```python
from build123d import *

# Parameters (mm, degrees)
SKETCH1_W            = 60
SKETCH1_H            = 45
BOSS_EXTRUDE1_DEPTH  = 5
SKETCH3_R            = 5.5
SKETCH3_R_2          = 3.025
BOSS_EXTRUDE2_DEPTH  = 8
SKETCH4_W            = 12
SKETCH4_H            = 16
SKETCH4_R            = 2.55
BOSS_EXTRUDE3_DEPTH  = 5
FILLET1_R            = 4
M4_CLEARANCE_HOLE1_D = 4.5
MIRROR1_OUTLINE_R    = 2.25
MIRROR1_DEPTH        = 5


# Read off the part's stored shape, not the designer's step: Mirror1
with BuildPart() as part:
    # Sketch1 → Boss-Extrude1 (new body)
    with BuildSketch(Plane.XY):
        Rectangle(SKETCH1_W, SKETCH1_H)
    extrude(amount=BOSS_EXTRUDE1_DEPTH)

    # Sketch3 → Boss-Extrude2 (add)
    # profile 1 of 4: a face of its own
    with BuildSketch(Plane.XY.offset(5)):
        with Locations((-19.2405, 11.938)):
            Circle(SKETCH3_R)
        with Locations((-19.2405, 11.938)):
            Circle(SKETCH3_R_2, mode=Mode.SUBTRACT)
    # profile 2 of 4: a face of its own
    with BuildSketch(Plane.XY.offset(5)):
        with Locations((-19.2405, -11.938)):
            Circle(SKETCH3_R)
        with Locations((-19.2405, -11.938)):
            Circle(SKETCH3_R_2, mode=Mode.SUBTRACT)
    # profile 3 of 4: a face of its own
    with BuildSketch(Plane.XY.offset(5)):
        with Locations((19.2405, 11.938)):
            Circle(SKETCH3_R)
        with Locations((19.2405, 11.938)):
            Circle(SKETCH3_R_2, mode=Mode.SUBTRACT)
    # profile 4 of 4: a face of its own
    with BuildSketch(Plane.XY.offset(5)):
        with Locations((19.2405, -11.938)):
            Circle(SKETCH3_R)
        with Locations((19.2405, -11.938)):
            Circle(SKETCH3_R_2, mode=Mode.SUBTRACT)
    extrude(amount=BOSS_EXTRUDE2_DEPTH)

    # Sketch4 → Boss-Extrude3 (add)
    # profile 1 of 2: a face of its own
    with BuildSketch(Plane.XY.offset(5)):
        with Locations((-36, 0)):
            Rectangle(SKETCH4_W, SKETCH4_H)
        with Locations((-36, 0)):
            Circle(SKETCH4_R, mode=Mode.SUBTRACT)
    # profile 2 of 2: a face of its own
    with BuildSketch(Plane.XY.offset(5)):
        with Locations((-36, 0)):
            Circle(SKETCH4_R)
    extrude(amount=-BOSS_EXTRUDE3_DEPTH)

    # Fillet1
    fillet1_edges = [part.edges().sort_by_distance(p)[0] for p in [
        (-42, -8, 2.5),
        (-42, 8, 2.5),
        (-30, 8, 2.5),
        (-30, -8, 2.5),
        (-30, 22.5, 2.5),
        (-30, -22.5, 2.5),
    ]]
    fillet(fillet1_edges, radius=FILLET1_R)

    # M4 Clearance Hole1 (through all)
    with Locations(Plane.XY.offset(5)):
        with Locations((-36, 0)):
            Hole(M4_CLEARANCE_HOLE1_D / 2)

    # Mirror1 outline → Mirror1 (add)
    with BuildSketch(Plane.XY):
        with BuildLine():
            ThreePointArc((42, 4), (40.828427125, 6.828427125), (38, 8))
            Line((38, 8), (30, 8))
            Line((30, 8), (30, -8))
            Line((30, -8), (38, -8))
            ThreePointArc((38, -8), (40.828427125, -6.828427125), (42, -4))
            Line((42, -4), (42, 4))
        make_face()
        with Locations((36, 0)):
            Circle(MIRROR1_OUTLINE_R, mode=Mode.SUBTRACT)
    extrude(amount=MIRROR1_DEPTH)


solid = part.part
```
The model under review builds one solid part; all positions refer to its coordinate system, in mm. A direction names the side the tool comes from. Give positions to 0.01 mm unless a question says otherwise; leave off trailing zeros. Write each loop counter-clockwise with the first axis right and the second up, starting at its lowest first coordinate (ties: lowest second). Pieces come first, ordered by that corner, then holes. Notation, with made-up numbers: M 86,-14 L 114,-14 A25 cw 114,-2 Z; hole C -4.5,62.25 d6. An arc over 180 degrees is marked long. Answer in a Markdown table with one row per item.
Item 1: Add section C-C on x = -36. Give the boundary of the cut face in (y, z).
Check sheet entries:
| item | result |
|---|---|
| outline | M -8,0 L -2.25,0 L -2.25,5 L -8,5 Z; M 2.25,0 L 8,0 L 8,5 L 2.25,5 Z |
Item 2: Add section D-D on z = 12. State how many separate pieces and enclosed holes the cut face has, plus the area to 3 significant figures.
Check sheet entries:
| item | result |
|---|---|
| separate pieces | 4 |
| enclosed holes | 4 |
| area | 265 mm2 |
Item 3: For P1, Ø3, axis at x = 19, y = 12.5, coming from the +Z side; P2, Ø2, axis at x = -36, z = 3.5, coming from the -Y side; P3, Ø1.5, axis at y = 14, z = 2.5, coming from the -X side, all flat-tipped, find the tip position at first contact; note any pin that passes through.
Check sheet entries:
| item | result |
|---|---|
| P1 | z = 5 |
| P2 | y = -8 |
| P3 | x = -30 |
Item 4: Tool access review of faces 4 (the face through (30, 15, 2)), 5 (the face through (14.876, 8.591, 8.944)), 6 (the face through (-36, 8, 3)), 7 (the face through (42, 0, 2)), 8 (the face through (34, -8, 2)): name each direction out of +Z, -Z, +X, -X, +Y, -Y from which nothing blocks a thin tool from reaching the whole face with its end or side.
Check sheet entries:
| item | result |
|---|---|
| face 4 | +Z, -Z, +X, +Y |
| face 5 | +Z |
| face 6 | +Z, -Z, -X, +Y |
| face 7 | +Z, -Z, +X, +Y, -Y |
| face 8 | +Z, -Z, +X, -Y |
Item 5: Draft analysis for pull direction Y (two halves, no side actions). For faces 1 (the face through (-20.433, -17.307, 8.944)), 2 (the face through (-30, 15, 2)), 3 (the face through (-40.859, 6.797, 2.465)), state which applies: +Y half, -Y half, draft (parallel to the pull), parting line (faces both ways), or undercut.
Check sheet entries:
| item | result |
|---|---|
| face 1 | undercut |
| face 2 | draft |
| face 3 | +Y half |
Item 6: Add section B-B on y = 0. Give the boundary of the cut face in (x, z), plus the area to 3 significant figures.
Check sheet entries:
| item | result |
|---|---|
| outline | M -42,0 L -38.25,0 L -38.25,5 L -42,5 Z; M -33.75,0 L 33.75,0 L 33.75,5 L -33.75,5 Z; M 38.25,0 L 42,0 L 42,5 L 38.25,5 Z |
| area | 375 mm2 |
Item 7: For line 1 along Y through (x, z) = (20, 6.5); line 2 along Y through (x, z) = (36, 2.6); line 3 along X through (y, z) = (-16, 9), list the stretches that pass through material, from the lowest coordinate up.
Check sheet entries:
| item | result |
|---|---|
| line 1 | -17.39 to -14.87, -9.01 to -6.49, 6.49 to 9.01, 14.87 to 17.39 |
| line 2 | -8 to -2.25, 2.25 to 8 |
| line 3 | -22.95 to -15.53, 15.53 to 22.95 |
Item 8: Add section A-A on z = 3.5. Give the boundary of the cut face in (x, y), plus the area to 3 significant figures.
Check sheet entries:
| item | result |
|---|---|
| outline | M -42,-4 A4 ccw -38,-8 L -34,-8 A4 cw -30,-12 L -30,-18.5 A4 ccw -26,-22.5 L 30,-22.5 L 30,-8 L 38,-8 A4 ccw 42,-4 L 42,4 A4 ccw 38,8 L 30,8 L 30,22.5 L -26,22.5 A4 ccw -30,18.5 L -30,12 A4 cw -34,8 L -38,8 A4 ccw -42,4 Z; hole C -36,0 d4.5; hole C 36,0 d4.5 |
| area | 3,040 mm2 |
